from build123d import *

# Parameters (mm, degrees)
CROQUIS1_R              = 31.5
SALIENTE_EXTRUIR1_DEPTH = 2.4
CROQUIS2_W              = 16.1
CROQUIS2_H              = 36.3
CROQUIS2_W_2            = 12.5
CROQUIS2_H_2            = 33
SALIENTE_EXTRUIR2_DEPTH = 22.5
CROQUIS5_W              = 16.1
CROQUIS5_H              = 36.3
CORTAR_EXTRUIR2_DEPTH   = 9
CROQUIS6_R              = 1.5
CORTAR_EXTRUIR3_DEPTH   = 2.4
CROQUIS7_W              = 12.5
CROQUIS7_H              = 9
SALIENTE_EXTRUIR3_DEPTH = 33
CROQUIS8_R              = 1
CORTAR_EXTRUIR5_DEPTH   = 9
SALIENTE_EXTRUIR4_DEPTH = 12.5
CROQUIS10_W             = 4
CROQUIS10_H             = 2
CORTAR_EXTRUIR6_DEPTH   = 9
SALIENTE_EXTRUIR5_DEPTH = 2.4
SALIENTE_EXTRUIR6_DEPTH = 16.099998
CORTAR_EXTRUIR7_DEPTH   = 1.8
CROQUIS14_R             = 1.5
SALIENTE_EXTRUIR7_DEPTH = 0.6
CORTAR_EXTRUIR8_START   = -17
CROQUIS17_R             = 41.453169239
CORTAR_EXTRUIR8_DEPTH   = 17


with BuildPart() as part:
    # Croquis1 → Saliente-Extruir1 (new body)
    with BuildSketch(Plane.XY):
        with Locations((-51.235671923, 9.786589019)):
            Circle(CROQUIS1_R)
    extrude(amount=SALIENTE_EXTRUIR1_DEPTH)

    # Croquis2 → Saliente-Extruir2 (add)
    with BuildSketch(Plane.XY.offset(2.4)):
        with Locations((-51.235671923, 4.936589019)):
            Rectangle(CROQUIS2_W, CROQUIS2_H)
        with Locations((-51.235671923, 4.786589019)):
            Rectangle(CROQUIS2_W_2, CROQUIS2_H_2, mode=Mode.SUBTRACT)
    extrude(amount=SALIENTE_EXTRUIR2_DEPTH)

    # Croquis5 → Cortar-Extruir2 (cut)
    with BuildSketch(Plane.XY.offset(2.4)):
        with Locations((-51.235671923, 4.936589019)):
            Rectangle(CROQUIS5_W, CROQUIS5_H)
    extrude(amount=-CORTAR_EXTRUIR2_DEPTH, mode=Mode.SUBTRACT)


with BuildPart() as cortar_extruir2_piece_1:
    # of the separate pieces the step leaves, piece 1, a body of its own (cortar_extruir2_pieces)
    add(part.part.solids().sort_by_distance((-19.735671923, 9.786589019, 0))[0])

    # Croquis6 → Cortar-Extruir3 (cut)
    with BuildSketch(Plane(origin=(0, 0, 0), x_dir=(-1, 0, 0), z_dir=(0, 0, -1))):
        with Locations((34.618662565, 26.403598377)):
            Circle(CROQUIS6_R)
        with Locations((67.85268128, 26.403598377)):
            Circle(CROQUIS6_R)
        with Locations((67.85268128, -6.830420339)):
            Circle(CROQUIS6_R)
        with Locations((34.618662565, -6.830420339)):
            Circle(CROQUIS6_R)
        Polygon((51.235671923, 23.086589019), (53.235671923, 23.086589019), (53.235671923, 43.086589019), (49.235671923, 43.086589019), (49.235671923, 23.086589019), align=None)
    extrude(amount=-CORTAR_EXTRUIR3_DEPTH, mode=Mode.SUBTRACT)



with BuildPart() as cortar_extruir2_piece_2:
    # of the separate pieces the step leaves, piece 2, a body of its own (cortar_extruir2_pieces)
    add(part.part.solids().sort_by_distance((-59.285671923, -13.213410981, 24.9))[0])

    # Croquis7 → Saliente-Extruir3 (add)
    with BuildSketch(Plane.XZ.offset(-21.286589019)):
        with Locations((-51.235671923, 13.4)):
            Rectangle(CROQUIS7_W, CROQUIS7_H)
    extrude(amount=SALIENTE_EXTRUIR3_DEPTH)

    # Croquis8 → Cortar-Extruir5 (cut)
    with BuildSketch(Plane.XY.offset(17.9)):
        with Locations((-51.235671923, -9.713410981)):
            Circle(CROQUIS8_R)
        with Locations((-51.235671923, 18.336589019)):
            Circle(CROQUIS8_R)
        Polygon((-44.985671923, -7.713410981), (-57.485671923, -7.713410981), (-57.485671923, 15.286589019), (-53.235671923, 15.286589019), (-53.235671923, 17.286589019), (-49.235671923, 17.286589019), (-49.235671923, 15.286589019), (-44.985671923, 15.286589019), align=None)
    extrude(amount=-CORTAR_EXTRUIR5_DEPTH, mode=Mode.SUBTRACT)

    # Croquis9 → Saliente-Extruir4 (add)
    with BuildSketch(Plane.ZY.offset(44.985671923)):
        Polygon((8.9, -7.713410981), (3.9, -11.713410981), (8.9, -11.713410981), align=None)
        Polygon((8.9, 15.286589019), (4.1, 21.286589019), (8.9, 21.286589019), align=None)
    extrude(amount=SALIENTE_EXTRUIR4_DEPTH)

    # Croquis10 → Cortar-Extruir6 (cut)
    with BuildSketch(Plane.XY.offset(8.9)):
        with Locations((-51.235671923, 16.286589019)):
            Rectangle(CROQUIS10_W, CROQUIS10_H)
    extrude(amount=-CORTAR_EXTRUIR6_DEPTH, mode=Mode.SUBTRACT)


with BuildPart() as cortar_extruir2_piece_1_1:
    add(cortar_extruir2_piece_1.part)

    add(cortar_extruir2_piece_2.part)  # Saliente-Extruir5 merges Cortar-Extruir2 piece 2
    # Croquis11 → Saliente-Extruir5 (add)
    with BuildSketch(Plane(origin=(0, 0, 2.4), x_dir=(-1, 0, 0), z_dir=(0, 0, -1))):
        Polygon((49.235671923, 23.086589019), (43.185671923, 23.086589019), (43.185671923, -13.213410981), (59.285671923, -13.213410981), (59.285671923, 23.086589019), (53.235671923, 23.086589019), (53.235671923, 21.286589019), (57.485671923, 21.286589019), (57.485671923, 10.586589019), (44.985671923, 10.586589019), (44.985671923, 21.286589019), (49.235671923, 21.286589019), align=None)
    extrude(amount=SALIENTE_EXTRUIR5_DEPTH)

    # Croquis12 → Saliente-Extruir6 (add)
    with BuildSketch(Plane(origin=(-43.185671923, 0, 0), x_dir=(0, 0, -1), z_dir=(1, 0, 0))):
        Polygon((-2.4, 23.086589019), (-7.4, 23.086589019), (-2.4, 29.386589019), align=None)
    extrude(amount=-SALIENTE_EXTRUIR6_DEPTH)

    # Croquis13 → Cortar-Extruir7 (cut)
    with BuildSketch(Plane.XY.offset(2.4)):
        Polygon((-31.385501057, -6.830420339), (-33.002081811, -4.030420339), (-36.235243318, -4.030420339), (-37.851824072, -6.830420339), (-36.235243318, -9.630420339), (-33.002081811, -9.630420339), align=None)
        Polygon((-64.619519773, -6.830420339), (-66.236100527, -4.030420339), (-69.469262034, -4.030420339), (-71.085842788, -6.830420339), (-69.469262034, -9.630420339), (-66.236100527, -9.630420339), align=None)
        Polygon((-37.851824072, 26.403598377), (-36.235243318, 23.603598377), (-33.002081811, 23.603598377), (-31.385501057, 26.403598377), (-33.002081811, 29.203598377), (-36.235243318, 29.203598377), align=None)
        Polygon((-71.085842788, 26.403598377), (-69.469262034, 23.603598377), (-66.236100527, 23.603598377), (-64.619519773, 26.403598377), (-66.236100527, 29.203598377), (-69.469262034, 29.203598377), align=None)
    extrude(amount=-CORTAR_EXTRUIR7_DEPTH, mode=Mode.SUBTRACT)

    # Croquis14 → Saliente-Extruir7 (add)
    with BuildSketch(Plane(origin=(0, 0, 0), x_dir=(-1, 0, 0), z_dir=(0, 0, -1))):
        with BuildLine():
            Line((53.235671923, 41.223032838), (53.235671923, 21.286589019))
            Line((53.235671923, 21.286589019), (57.485671923, 21.286589019))
            Line((57.485671923, 21.286589019), (57.485671923, 10.586589019))
            Line((57.485671923, 10.586589019), (44.985671923, 10.586589019))
            Line((44.985671923, 10.586589019), (44.985671923, 21.286589019))
            Line((44.985671923, 21.286589019), (49.235671923, 21.286589019))
            Line((49.235671923, 21.286589019), (49.235671923, 41.223032838))
            ThreePointArc((49.235671923, 41.223032838), (51.235671923, -21.713410981), (53.235671923, 41.223032838))
        make_face()
        with Locations((67.85268128, -6.830420339)):
            Circle(CROQUIS14_R, mode=Mode.SUBTRACT)
        with Locations((34.618662565, -6.830420339)):
            Circle(CROQUIS14_R, mode=Mode.SUBTRACT)
        with Locations((34.618662565, 26.403598377)):
            Circle(CROQUIS14_R, mode=Mode.SUBTRACT)
        with Locations((67.85268128, 26.403598377)):
            Circle(CROQUIS14_R, mode=Mode.SUBTRACT)
    extrude(amount=SALIENTE_EXTRUIR7_DEPTH)

    # Croquis17 → Cortar-Extruir8 (cut)
    with BuildSketch(Plane.XY.offset(16.4).offset(CORTAR_EXTRUIR8_START)):
        with Locations((-51.749775456, 10.131791007)):
            Circle(CROQUIS17_R)
    extrude(amount=CORTAR_EXTRUIR8_DEPTH, mode=Mode.SUBTRACT)


solid = cortar_extruir2_piece_1_1.part
For this review, take the finished solid that the model builds, in its own axes (mm). A direction names the side the tool comes from. Coordinates: 2 decimals unless noted, no trailing zeros. Order: outer loops, then holes, each group sorted by start corner. A loop starts at its lowest first (then second) coordinate and runs counter-clockwise, first axis right, second up. Notation, with made-up numbers: (46.25, 36.25) - (85.25, 36.25) arc R17 ccw to (85.25, 67.25) - close; hole circle Ø1 at (-32.5, 20.25). An arc over 180 degrees is marked (long way). Use one line per item in the form item = value.
Q1. Draft analysis for pull direction X (two halves, no side actions). For faces 1 (the flat face through (-55, 15.287, 17)), 2 (the flat face through (-43.186, 5, 21)), 3 (the flat face through (-51, 23.087, 21)), state which applies: +X half, -X half, draft (parallel to the pull), parting line (faces both ways), or undercut.
Checked values:
face_1 = undercut
face_2 = +X half
face_3 = draft
Q2. For faces 4 (the flat face through (-59, 9, 16.4)), 5 (the flat face through (-51, -11.713, 21)), 6 (the flat face through (-53.236, 16, 17)), list the 3-axis set-ups (+Z, -Z, +X, -X, +Y, -Y) from which the entire face can be reached by the end or side of a thin tool; tool diameter is ignored.
Checked values:
face_4 = -Z, +X, -X, +Y, -Y
face_5 = +Z
face_6 = +Z, -Z
Q3. Consider section C-C (z = 19.5). Give the boundary of the cut face in (x, y).
Checked values:
outline = (-59.29, -13.21) - (-43.19, -13.21) - (-43.19, 23.09) - (-59.29, 23.09) - close; hole (-57.49, -11.71) - (-44.99, -11.71) - (-44.99, 21.29) - (-57.49, 21.29) - close
Q4. Consider section B-B (y = 4.5). Give the boundary of the cut face in (x, z).
Checked values:
outline = (-59.29, 16.4) - (-57.49, 16.4) - (-57.49, 24.9) - (-59.29, 24.9) - close; (-44.99, 16.4) - (-43.19, 16.4) - (-43.19, 24.9) - (-44.99, 24.9) - close
Q5. For P1, Ø1.2, axis at x = -51.24, y = -9.71, coming from the -Z side; P2, Ø3, axis at x = -53, y = 19.5, coming from the +Z side, all flat-tipped, find the tip position at first contact; note any pin that passes through.
Checked values:
P1 = through
P2 = 17.9
Q6. Consider section A-A (x = -47.25). Give the boundary of the cut face in (y, z).
Checked values:
outline = (-13.21, 16.4) - (-7.71, 16.4) - (-7.71, 17.9) - (-11.71, 17.9) - (-11.71, 24.9) - (-13.21, 24.9) - close; (15.29, 16.4) - (23.09, 16.4) - (23.09, 24.9) - (21.29, 24.9) - (21.29, 17.9) - (15.29, 17.9) - close
Q7. For probe 1 along X at (y, z) = (12, 22); probe 2 along Y at (x, z) = (-50.5, 18.5); probe 3 along Z at (x, y) = (-56.75, 20), list the stretches that pass through material, from the lowest coordinate up. Write a range as from..to.
Checked values:
probe_1 = -59.29..-57.49, -44.99..-43.19
probe_2 = -13.21..-11.71, 21.29..23.09
probe_3 = 16.4..17.9
